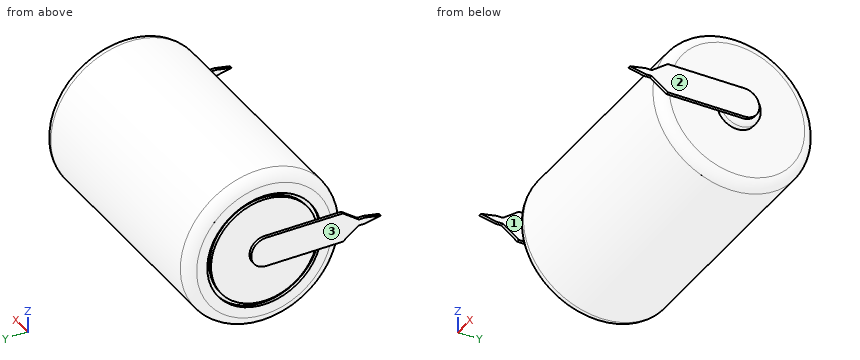
```python
from build123d import *

# Parameters (mm, degrees)
SKETCH1_R           = 7.5
BOSS_EXTRUDE1_DEPTH = 24
FILLET1_R           = 1
SKETCH2_R           = 1.924270806
BOSS_EXTRUDE2_DEPTH = 1
FILLET2_R           = 0.5
SKETCH3_R           = 5.477488552
SKETCH3_R_2         = 5.118293918
CUT_EXTRUDE1_DEPTH  = 0.3
BOSS_EXTRUDE3_DEPTH = 0.3
BOSS_EXTRUDE4_START = 0.3
BOSS_EXTRUDE4_DEPTH = 0.3


with BuildPart() as part:
    # Sketch1 → Boss-Extrude1 (new body)
    with BuildSketch(Plane(origin=(0, 0, 0), x_dir=(0, 0, -1), z_dir=(1, 0, 0))):
        Circle(SKETCH1_R)
    extrude(amount=BOSS_EXTRUDE1_DEPTH)

    # Fillet1
    fillet1_edges = [part.edges().sort_by_distance(p)[0] for p in [
        (0, 0, 7.5),
        (24, 0, 7.5),
    ]]
    fillet(fillet1_edges, radius=FILLET1_R)

    # Sketch2 → Boss-Extrude2 (add)
    with BuildSketch(Plane(origin=(24, 0, 0), x_dir=(0, 0, -1), z_dir=(1, 0, 0))):
        Circle(SKETCH2_R)
    extrude(amount=BOSS_EXTRUDE2_DEPTH)

    # Fillet2
    fillet2_edges = [part.edges().sort_by_distance(p)[0] for p in [
        (25, 0, 1.924270806),
    ]]
    fillet(fillet2_edges, radius=FILLET2_R)

    # Sketch3 → Cut-Extrude1 (cut)
    with BuildSketch(Plane.ZY):
        Circle(SKETCH3_R)
        Circle(SKETCH3_R_2, mode=Mode.SUBTRACT)
    extrude(amount=-CUT_EXTRUDE1_DEPTH, mode=Mode.SUBTRACT)

    # Sketch4 → Boss-Extrude3 (add)
    with BuildSketch(Plane(origin=(25, 0, 0), x_dir=(0, 0, -1), z_dir=(1, 0, 0))):
        with BuildLine():
            Line((-1.424270806, 0), (-1.424270806, -7.363521757))
            Line((-1.424270806, -7.363521757), (-0.511928366, -8.610369315))
            Line((-0.511928366, -8.610369315), (-0.3, -8.9))
            Line((-0.3, -8.9), (-0.3, -9.5))
            Line((-0.3, -9.5), (0, -11))
            Line((0, -11), (0.3, -9.5))
            Line((0.3, -9.5), (0.3, -8.9))
            Line((0.3, -8.9), (0.520522804, -8.598623776))
            Line((0.520522804, -8.598623776), (1.424270806, -7.363521757))
            Line((1.424270806, -7.363521757), (1.424270806, 0))
            ThreePointArc((1.424270806, 0), (0, 1.424270806), (-1.424270806, 0))
        make_face()
    extrude(amount=BOSS_EXTRUDE3_DEPTH)

    # Sketch5 → Boss-Extrude4 (add)
    with BuildSketch(Plane.ZY.offset(BOSS_EXTRUDE4_START)):
        with BuildLine():
            Line((-0.3, -8.9), (-0.3, -9.5))
            Line((-0.3, -9.5), (0, -11))
            Line((0, -11), (0.3, -9.5))
            Line((0.3, -9.5), (0.3, -8.9))
            Line((0.3, -8.9), (0.511928366, -8.610369315))
            Line((0.511928366, -8.610369315), (1.424270806, -7.363521757))
            Line((1.424270806, -7.363521757), (1.424270806, 0))
            ThreePointArc((1.424270806, 0), (0, 1.424270806), (-1.424270806, 0))
            Line((-1.424270806, 0), (-1.424270806, -7.363521757))
            Line((-1.424270806, -7.363521757), (-0.520522804, -8.598623776))
            Line((-0.520522804, -8.598623776), (-0.3, -8.9))
        make_face()
    extrude(amount=-BOSS_EXTRUDE4_DEPTH)


solid = part.part
```
Part model, mm, in its own coordinate system. Face numbers are marked on the shaded views. Coordinates: 2 decimals unless noted, no trailing zeros. Order: outer loops, then holes, each group sorted by start corner. A loop starts at its lowest first (then second) coordinate and runs counter-clockwise, first axis right, second up. Notation, with made-up numbers: (44.25, 46.25) -> (97.25, 46.25) arc R17 cw to (97.25, 59.25) -> close; hole circle Ø1 at (36.25, 71.5). An arc over 180 degrees is marked (long way). Put each result on its own line as item: value. Start each with the question number.
(1) Probe line 1 along Y through (x, z) = (0.2, 0); line 2 along Y through (x, z) = (6, -0.25); line 3 along X through (y, z) = (1, -3.5). List the from-to ranges inside material, lowest first. Write a range as [from, to].
(2) Mould opens along X. For the marked faces 1, 2 and 3 say: pulls with the +X half, pulls with the -X half, needs draft (parallel to the pull), parting line crosses it, or undercut.
(3) Band-saw the part on A-A (y = -10). Give the cut face in (x, z).
(4) Band-saw the part on B-B (x = 10). Give the cut face in (y, z).
(5) Pin check, flat tips, straight feed: pin 1 Ø1 at (x, z) = (13, -2.5) entering from -Y; pin 2 Ø6 at (x, y) = (22, 4.5) entering from +Z; pin 3 Ø1.5 at (x, z) = (22, -4) entering from +Y. Stop position of each tip, or through.
Determined:
1. line 1: y = [-7.1, -5.48], [-5.12, 5.12], [5.48, 7.1]
1. line 2: y = [-7.5, 7.5]
1. line 3: x = [0, 24]
2. face 1: undercut
2. face 2: pulls with the +X half
2. face 3: pulls with the -X half
3. outline: (-0.3, -0.2) -> (0, -0.2) -> (0, 0.2) -> (-0.3, 0.2) -> close; (25, -0.2) -> (25.3, -0.2) -> (25.3, 0.2) -> (25, 0.2) -> close
4. outline: circle Ø15 at (0, 0)
5. pin 1: stops at y = -7.23
5. pin 2: stops at z = 7.35
5. pin 3: stops at y = 6.76
